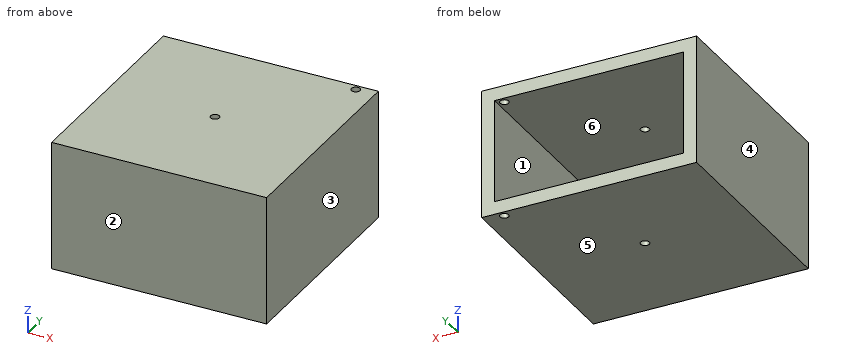
from build123d import *

# Parameters (mm, degrees)
SKETCH1_W           = 250
SKETCH1_H           = 250
BOSS_EXTRUDE1_DEPTH = 150
SKETCH2_W           = 220
SKETCH2_H           = 120
CUT_EXTRUDE1_DEPTH  = 235
SKETCH3_R           = 5
CUT_EXTRUDE5_DEPTH  = 235


with BuildPart() as part:
    # Sketch1 → Boss-Extrude1 (new body)
    with BuildSketch(Plane.XY):
        with Locations((125, -125)):
            Rectangle(SKETCH1_W, SKETCH1_H)
    extrude(amount=BOSS_EXTRUDE1_DEPTH)

    # Sketch2 → Cut-Extrude1 (cut)
    with BuildSketch(Plane(origin=(0, 0, 0), x_dir=(1, 0, 0), z_dir=(0, 1, 0))):
        with Locations((125, -75)):
            Rectangle(SKETCH2_W, SKETCH2_H)
    extrude(amount=-CUT_EXTRUDE1_DEPTH, mode=Mode.SUBTRACT)

    # Sketch3 → Cut-Extrude5 (cut)
    with BuildSketch(Plane.XY.offset(150)):
        with Locations((125, -125)):
            Circle(SKETCH3_R)
        with Locations((227.5, -7.5)):
            Circle(SKETCH3_R)
    extrude(amount=-CUT_EXTRUDE5_DEPTH, mode=Mode.SUBTRACT)


solid = part.part
Design review of the part built by this model. Coordinates are the model's own, in mm. Face numbers are marked on the shaded views. A direction names the side the tool comes from. Give positions to 0.01 mm unless a question says otherwise; leave off trailing zeros. Order: outer loops, then holes, each group sorted by start corner. A loop starts at its lowest first (then second) coordinate and runs counter-clockwise, first axis right, second up. Notation, with made-up numbers: (86, 77.25) - (129, 77.25) arc R23 ccw to (129, 103.25) - close; hole circle Ø10 at (49, -37). An arc over 180 degrees is marked (long way). Write item = value, one per line. Start each with the question number.
Q1. We need section A-A on y = -125. State the section outline as (x, z) points.
Q2. We need section B-B on x = 227.5. State the section outline as (y, z) points.
Q3. Mouldability with a two-part tool opening along X and no side actions: class the marked faces 3, 4, 5 and 6 as released by +X, released by -X, zero draft, split by the parting line, or undercut.
Q4. Clearance check with flat-ended pins moving along their axes: pin 1 Ø11.5 at (x, y) = (227.5, -7.5) entering from -Z; pin 2 Ø3 at (x, z) = (117.5, 103.5) entering from +Y. State where each tip first meets the part, or that it passes through.
Q5. Tool access review of the marked faces 1 and 2: name each direction out of +Z, -Z, +X, -X, +Y, -Y from which nothing blocks a thin tool from reaching the whole face with its end or side.
Q6. We need section C-C on y = -92. State the section outline as (x, z) points, plus the area to 3 significant figures.
Q7. We need section D-D on z = 86.5. State the section outline as (x, y) points, plus the area to 3 significant figures.
Q8. To check wall thickness, follow L1, parallel to Z at x = 59, y = -117.5; L2, parallel to X at y = -60, z = 55; L3, parallel to Y at x = 125, z = 144. State the ranges of each line that lie inside material, in increasing order. Write a range as from..to.
Working result:
q1.outline = (0, 0) - (120, 0) - (120, 15) - (15, 15) - (15, 135) - (120, 135) - (120, 150) - (0, 150) - close; (130, 0) - (250, 0) - (250, 150) - (130, 150) - (130, 135) - (235, 135) - (235, 15) - (130, 15) - close
q2.outline = (-250, 0) - (-12.5, 0) - (-12.5, 15) - (-235, 15) - (-235, 135) - (-12.5, 135) - (-12.5, 150) - (-250, 150) - close; (-2.5, 0) - (0, 0) - (0, 15) - (-2.5, 15) - close; (-2.5, 135) - (0, 135) - (0, 150) - (-2.5, 150) - close
q3.face_3 = released by +X
q3.face_4 = released by -X
q3.face_5 = zero draft
q3.face_6 = undercut
q4.pin_1 = 0
q4.pin_2 = -235
q5.face_1 = +Y
q5.face_2 = +Z, -Z, +X, -X, -Y
q6.outline = (0, 0) - (250, 0) - (250, 150) - (0, 150) - close; hole (15, 15) - (235, 15) - (235, 135) - (15, 135) - close
q6.area = 11,100 mm²
q7.outline = (0, -250) - (250, -250) - (250, 0) - (235, 0) - (235, -235) - (15, -235) - (15, 0) - (0, 0) - close
q7.area = 10,800 mm²
q8.L1 = 0..15, 135..150
q8.L2 = 0..15, 235..250
q8.L3 = -250..-130, -120..0
